Autodesk Fusion 360 part; units mm, degrees
sketch "sketch 237" plane through (0, -32.5, 0) normal (0, -1, 0) x (1, 0, 0)
  line L0 (-84, 110) -> (-109, 105)
  line L1 (-109, 105) -> (-109, 102.5)
  line L2 (-109, 102.5) -> (11, 102.5)
  line L3 (11, 102.5) -> (11, 120)
  line L4 (11, 120) -> (1, 120)
  line L5 (1, 120) -> (1, 110)
  line L6 (1, 110) -> (-84, 110)
  line L7 (0.5, 110.5) -> (-19.5, 110.5)
  line L8 (-19.5, 110.5) -> (-19.5, 135)
  line L9 (-19.5, 135) -> (0.5, 135)
  line L10 (0.5, 135) -> (0.5, 110.5)
  line L11 (0.5, 135) -> (11, 135)
  line L12 (11, 135) -> (11, 121)
  line L13 (11, 121) -> (0.5, 121)
  line L14 (0.5, 121) -> (0.5, 135)
  dimension "d50" = 0.5
  dimension "d51" = 0.5
  dimension "d52" = 15
  dimension "d53" = 20
  dimension "d54" = 1
extrude "Extrude1" add sketch "sketch 237" against normal blind 90 contours L7 L8 L9 L10 L14 | L10 L11 L12 L13 L14
sketch "sketch 690" plane through (0, 0, 135) normal (0, 0, 1) x (-1, 0, 0)
  line L0 (-10, -39) -> (-11, -40)
  line L1 (-11, -40) -> (-11, -47.5)
  line L2 (-11, -47.5) -> (-1, -57.5)
  line L3 (-1, -57.5) -> (9.5, -57.5)
  line L4 (9.5, -57.5) -> (9.5, 32.5)
  line L5 (9.5, 32.5) -> (-1, 32.5)
  line L6 (-1, 32.5) -> (-11, 22.5)
  line L7 (-11, 22.5) -> (-11, 15)
  line L8 (-11, 15) -> (-10, 14)
  line L9 (-10, 14) -> (-8, 14)
  line L10 (-8, 14) -> (-8, 5.5)
  line L11 (-8, 5.5) -> (-10, 5.5)
  line L12 (-10, 5.5) -> (-11, 4.5)
  line L13 (-11, 4.5) -> (-11, -29.5)
  line L14 (-11, -29.5) -> (-10, -30.5)
  line L15 (-10, -30.5) -> (-8, -30.5)
  line L16 (-8, -30.5) -> (-8, -39)
  line L17 (-8, -39) -> (-10, -39)
  line L18 (-11, -12.5) -> (-22, -12.5) construction
  line L19 (-22, -12.5) -> (-22, -25) construction
  line L20 (-22, -25) -> (-11, -25)
  line L21 (-22, 0) -> (-11, 0)
  line L22 (-22, -12.5) -> (-22, 0) construction
  arc A0 (-22, 0) -> (-22, -25) centre (-22, -12.5) ccw
  dimension "d66" = 11
  dimension "d67" = 12.5
extrude "Extrude3" add sketch "sketch 690" against normal up to surface (14 mm away) contours L13 L20 L21 A0
sketch "sketch 1375" plane through (0.5, 57.5, -0.7504) normal (0, 1, 0) x (-1, 0, 0)
  line L0 (2, 111.2504) -> (5, 111.2504)
  line L1 (2, 111.2504) -> (5, 111.2504)
  line L2 (2, 111.2504) -> (5, 111.2504)
  line L3 (5, 111.2504) -> (0, 121.7504)
  line L4 (0, 121.7504) -> (0, 113.2504)
  line L5 (0, 121.7504) -> (0, 113.2504)
  line L6 (0, 121.7504) -> (0, 113.2504)
  line L7 (0, 113.2504) -> (2, 111.2504)
  line L8 (0, 113.2504) -> (2, 111.2504)
  line L9 (0, 113.2504) -> (2, 111.2504)
extrude "Extrude4" cut sketch "sketch 1375" against normal blind 6
Work out the finished part from the listing and answer in its coordinate system (mm). A direction names the side the tool comes from. Give positions to 0.01 mm unless a question says otherwise; leave off trailing zeros. Loops run counter-clockwise (first coordinate to the right, second up) from the corner with the lowest first, then second, coordinate; pieces in that order, holes last. Notation, with made-up numbers: (-16, -30.75) - (41, -30.75) arc R17 ccw to (41, -15.75) - close; hole circle Ø5 at (39.25, -26). An arc over 180 degrees is marked (long way). Answer in a Markdown table with one row per item. Add a question column.
Q1. The part is cut by section D-D (y = 12.5). Determine the outline of the cut face in (x, z), and give its area (3 significant figures).
Q2. The part is cut by section C-C (x = 20). Determine the outline of the cut face in (y, z), and give its area (3 significant figures).
Q3. The part is cut by section B-B (y = 36.5). Determine the outline of the cut face in (x, z), and give its area (3 significant figures).
Q4. Consider line 1 along X through (y, z) = (29.5, 126.25); line 2 along Z through (x, y) = (3.5, -10); line 3 along X through (y, z) = (10, 115.75). Determine where each line is inside the solid, lowest interval first.
Q5. A tool of negligible diameter and unlimited length cuts with its end or side. For faces 4 (the flat face through (11, -16, 128)), 5 (the flat face through (17, 25, 128)), 6 (the flat face through (-19.5, 12, 123)), 7 (the flat face through (0.5, 12, 116)), 8 (the flat face through (0, 55, 112)), from which of +Z, -Z, +X, -X, +Y, -Y can it reach the whole face along a straight path? Write none if from no direction.
Q6. Each of these flat-tipped pins is pushed along its axis until it touches: P1, Ø1.5, axis at y = 6, z = 131, coming from the +X side; P2, Ø8.5, axis at y = 33, z = 118, coming from the +X side; P3, Ø12, axis at y = 25.5, z = 123, coming from the +X side; P4, Ø12, axis at x = 14.5, z = 125, coming from the -Y side. Where does it stop, or does it pass through?
Q7. Determine the mould class of faces 1 (the flat face through (-1, 51.5, 113)), 2 (the flat face through (-8, 57.5, 126)), 3 (the flat face through (10, 12, 121)) for opening direction Z: released by +Z, released by -Z, zero draft, split by the parting line, or undercut.
Q8. The part is cut by section A-A (z = 125.5). Determine the outline of the cut face in (x, y), and give its area (3 significant figures).
Solution:
| question | item | result |
|---|---|---|
| 1 | outline | (-19.5, 110.5) - (0.5, 110.5) - (0.5, 121) - (34.5, 121) - (34.5, 135) - (-19.5, 135) - close |
| 1 | area | 966 mm² |
| 2 | outline | (0, 121) - (25, 121) - (25, 135) - (0, 135) - close |
| 2 | area | 350 mm² |
| 3 | outline | (-19.5, 110.5) - (0.5, 110.5) - (0.5, 121) - (11, 121) - (11, 135) - (-19.5, 135) - close |
| 3 | area | 637 mm² |
| 4 | line 1 | x = -19.5 to 11 |
| 4 | line 2 | z = 121 to 135 |
| 4 | line 3 | x = -19.5 to 0.5 |
| 5 | face 4 | +Z, -Z, +X, -Y |
| 5 | face 5 | +Z, -Z, +X, +Y |
| 5 | face 6 | +Z, -Z, -X, +Y, -Y |
| 5 | face 7 | -Z, +X, +Y, -Y |
| 5 | face 8 | +Y |
| 6 | P1 | stops at x = 33.1 |
| 6 | P2 | stops at x = 11 |
| 6 | P3 | stops at x = 32.36 |
| 6 | P4 | stops at y = -32.5 |
| 7 | face 1 | undercut |
| 7 | face 2 | zero draft |
| 7 | face 3 | released by -Z |
| 8 | outline | (-19.5, -32.5) - (11, -32.5) - (11, 0) - (22, 0) arc R12.5 ccw to (22, 25) - (11, 25) - (11, 57.5) - (-19.5, 57.5) - close |
| 8 | area | 3,270 mm² |
